Geometry: see drawing. Coordinates: mm, zero at the bounding-box minimum. Give positions to 0.01 mm unless a question says otherwise; leave off trailing zeros. Loops run counter-clockwise (first coordinate to the right, second up) from the corner with the lowest first, then second, coordinate; pieces in that order, holes last. Notation, with made-up numbers: M 62.25,-13 L 77.25,-13 A28 cw 77.25,6 Z; hole C 73.25,60 d4. An arc over 180 degrees is marked long. Put each result on its own line as item: value.
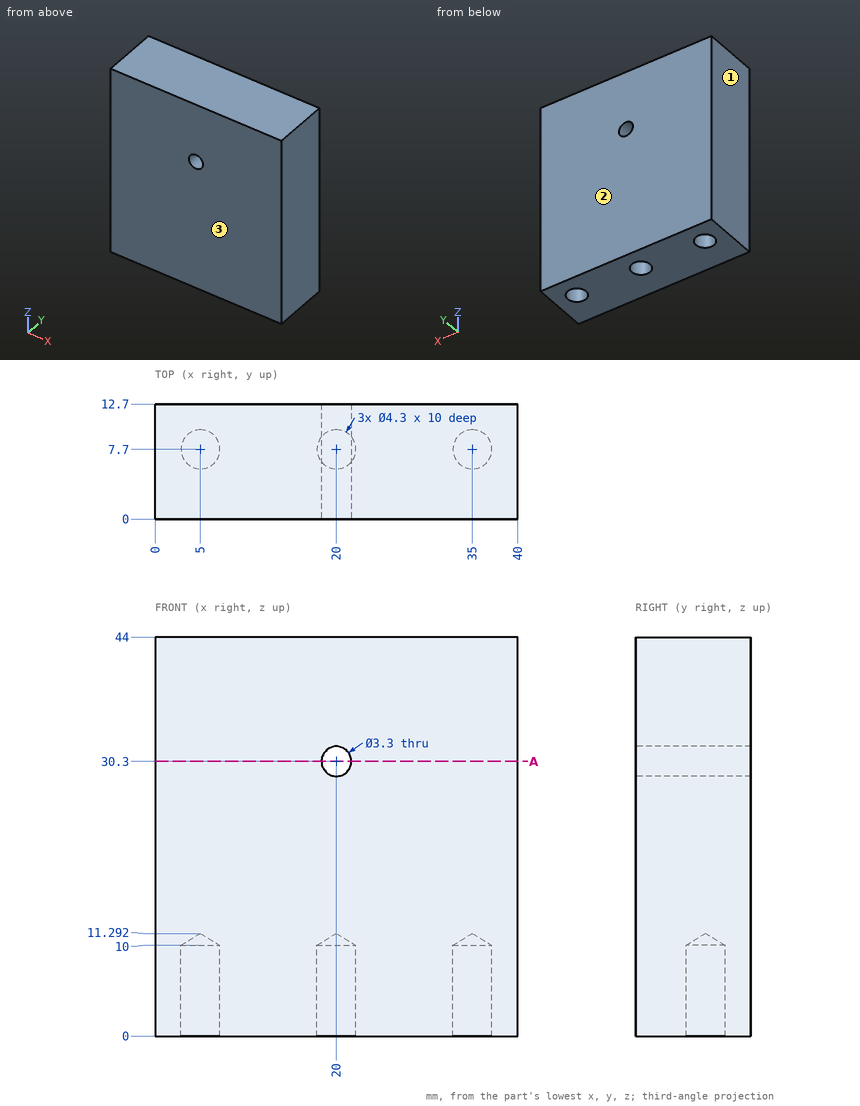
Item 1: Line query: probe 1 along X at (y, z) = (7.7, 8.25); probe 2 along Y at (x, z) = (5, 7); probe 3 along Z at (x, y) = (20.5, 2.25). Output: solid intervals per line, ascending. Write a range as [from, to].
Output values:
probe 1: [0, 2.85], [7.15, 17.85], [22.15, 32.85], [37.15, 40]
probe 2: [0, 5.55], [9.85, 12.7]
probe 3: [0, 28.73], [31.87, 44]
Item 2: Mould query, pull axis Y, two halves, no side actions, for the marked faces 1, 2 and 3. Classes: pulls with the +Y half, pulls with the -Y half, needs draft (parallel to the pull), parting line crosses it, or undercut.
Output values:
face 1: needs draft
face 2: pulls with the +Y half
face 3: pulls with the -Y half
Item 3: Section A-A on z = 30.3. Output: boundary loops of the cut face in (x, y).
Output values:
outline: M 0,0 L 18.35,0 L 18.35,12.7 L 0,12.7 Z; M 21.65,0 L 40,0 L 40,12.7 L 21.65,12.7 Z
Item 4: Pin query (flat end, axial travel): pin 1 Ø3.5 at (x, y) = (20, 7.7) entering from -Z; pin 2 Ø2 at (x, z) = (20, 30.3) entering from -Y; pin 3 Ø2.5 at (x, y) = (5, 7.7) entering from -Z. Return the tip coordinate at first contact, or that it passes through.
Output values:
pin 1: z = 10.24
pin 2: through
pin 3: z = 10.54
